Part print with two shaded views. Sizes in mm from the minimum x, y, z corner. A direction names the side the tool comes from. Give positions to 0.01 mm unless a question says otherwise; leave off trailing zeros. Order: outer loops, then holes, each group sorted by start corner. A loop starts at its lowest first (then second) coordinate and runs counter-clockwise, first axis right, second up. Notation, with made-up numbers: M 79.5,32 L 97.5,32 A9 ccw 97.5,46 Z; hole C 79,78.25 d6. An arc over 180 degrees is marked long. Return JSON: item names as keys, results as strings.
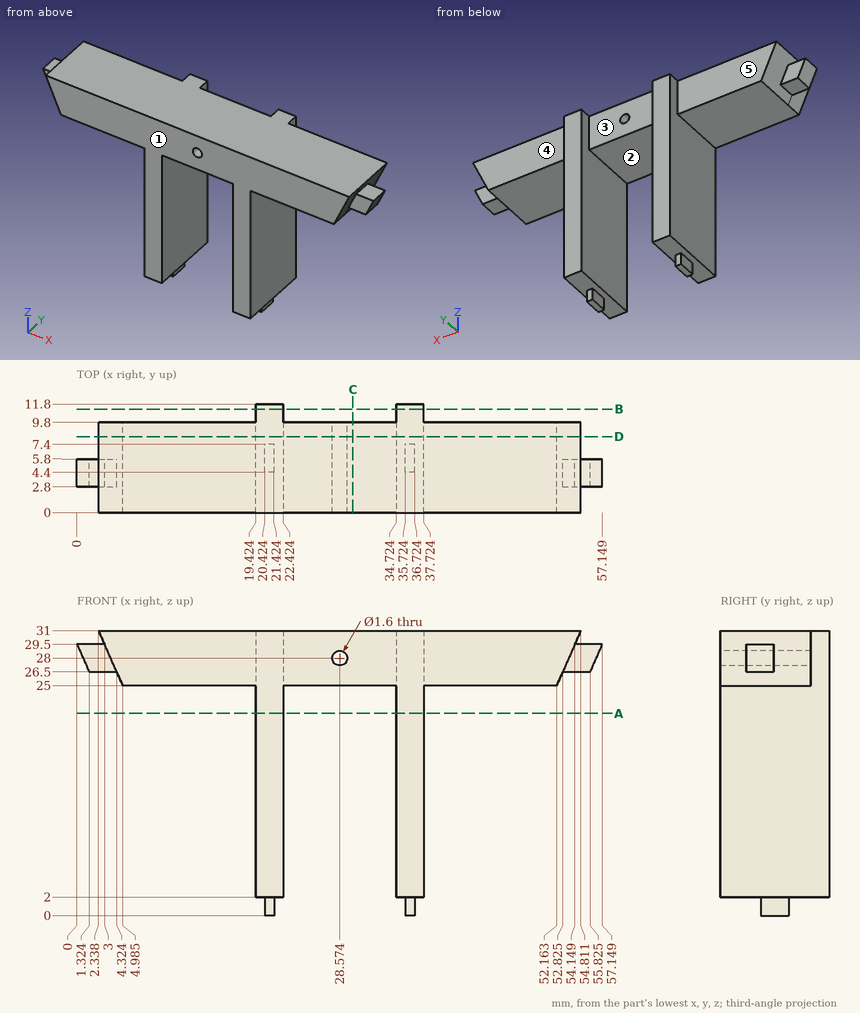
Q1. Band-saw the part on C-C (x = 30). Give the cut face in (y, z), then the cut area to 3 significant figures.
Established:
{"outline": "M 0,25 L 9.8,25 L 9.8,31 L 0,31 Z", "area": "58.8 mm²"}
Q2. Pin check, flat tips, straight feed: pin 1 (1.3 mm diameter, centred on x = 28.57, z = 28, fed in from +Y); pin 2 (0.9 mm diameter, centred on x = 1.5, y = 4.5, fed in from +Z); pin 3 (2 mm diameter, centred on y = 8, z = 3.5, fed in from -X); pin 4 (0.9 mm diameter, centred on x = 55, z = 27.5, fed in from -Y). Stop position of each tip, or through.
Established:
{"pin 1": "passes through", "pin 2": "stops at z = 29.5", "pin 3": "stops at x = 19.42", "pin 4": "stops at y = 2.8"}
Q3. Two-plate mould, pull along X, no slides. Class the marked faces 1 and 2: +X half, -X half, draft (parallel to the pull), parting line (faces both ways), or undercut.
Established:
{"face 1": "draft", "face 2": "undercut"}
Q4. Band-saw the part on B-B (y = 11.25). Give the cut face in (x, z) (1 decimal), then the cut area to 3 significant figures.
Established:
{"outline": "M 19.4,2 L 22.4,2 L 22.4,31 L 19.4,31 Z; M 34.7,2 L 37.7,2 L 37.7,31 L 34.7,31 Z", "area": "174 mm²"}
Q5. Band-saw the part on A-A (z = 22). Give the cut face in (x, y) (1 decimal).
Established:
{"outline": "M 19.4,0 L 22.4,0 L 22.4,11.8 L 19.4,11.8 Z; M 34.7,0 L 37.7,0 L 37.7,11.8 L 34.7,11.8 Z"}
Q6. 3-axis set-ups, long thin cutter, end or side, ignore diameter. For the marked faces 3, 4 and 5: which of +Z, -Z, +X, -X, +Y, -Y reach the whole face in a straight line?
Established:
{"face 3": "+Z, -Z, +Y", "face 4": "+Z, -Z, +X, +Y", "face 5": "+Z, -Z, -X, +Y"}
Q7. Band-saw the part on D-D (y = 8.25). Give the cut face in (x, z) (1 decimal), then the cut area to 3 significant figures.
Established:
{"outline": "M 2.3,31 L 5,25 L 19.4,25 L 19.4,2 L 22.4,2 L 22.4,25 L 34.7,25 L 34.7,2 L 37.7,2 L 37.7,25 L 52.2,25 L 54.8,31 Z; hole C 28.6,28 d1.6", "area": "435 mm²"}
Q8. Probe line 1 along X through (y, z) = (5, 8) (1 decimal); line 2 along Z through (x, y) = (9.5, 1.75); line 3 along X through (y, z) = (7.75, 28) (1 decimal). List the from-to ranges inside material, lowest first.
Established:
{"line 1": "x = 19.4 to 22.4, 34.7 to 37.7", "line 2": "z = 25 to 31", "line 3": "x = 3.7 to 27.8, 29.4 to 53.5"}
